```python
from build123d import *

# Parameters (mm, degrees)
SKETCH_1_R               = 1.65
SKETCH_1_R_2             = 9
EXTRUDE_1_DEPTH          = 3
SKETCH_2_R               = 15.5
SKETCH_2_R_2             = 9
EXTRUDE_2_DEPTH          = 7
SKETCH_3_W               = 2.5
SKETCH_3_H               = 20
CUT_EXTRUDE_1_DEPTH      = 28
CUT_EXTRUDE_2_DEPTH      = 44.016618519
CUT_EXTRUDE_2_DEPTH_BACK = 44.016618519
SKETCH_4_R               = 1.1
SKETCH_5_R               = 10
CUT_EXTRUDE_3_DEPTH      = 43.210780613
SKETCH_6_R               = 1.9
CUT_EXTRUDE_8_DEPTH      = 13
CHAMFER_1_SIZE           = 2
FILLET_2_R               = 2
SKETCH_7_R               = 4
SKETCH_7_R_2             = 1.65
EXTRUDE_3_DEPTH          = 2
FILLET_3_R               = 0.5


with BuildPart() as part:
    # 草图1 → 凸台-拉伸1 (new body)
    with BuildSketch(Plane.XY):
        Polygon((0, 31), (-26.846787517, -15.5), (26.846787517, -15.5), align=None)
        with Locations((0, 20)):
            Circle(SKETCH_1_R, mode=Mode.SUBTRACT)
        with Locations((17.320508076, -10)):
            Circle(SKETCH_1_R, mode=Mode.SUBTRACT)
        with Locations((-17.320508076, -10)):
            Circle(SKETCH_1_R, mode=Mode.SUBTRACT)
        Circle(SKETCH_1_R_2, mode=Mode.SUBTRACT)
    extrude(amount=EXTRUDE_1_DEPTH)

    # 草图2 → 凸台-拉伸2 (add)
    with BuildSketch(Plane.XY.offset(3)):
        with Locations(Location((0, 0, 0), (0, 0, 150))):
            Circle(SKETCH_2_R)
        Circle(SKETCH_2_R_2, mode=Mode.SUBTRACT)
    extrude(amount=EXTRUDE_2_DEPTH)

    # 草图3 → 切除-拉伸1 (cut)
    with BuildSketch(Plane.XY.offset(10)):
        with Locations((0, -9)):
            Rectangle(SKETCH_3_W, SKETCH_3_H)
    extrude(amount=-CUT_EXTRUDE_1_DEPTH, mode=Mode.SUBTRACT)

    # 草图4 → 切除-拉伸2 (cut, two sides: drawn at the far end of the back side and taken through both)
    with BuildSketch(Plane(origin=(-1.25, 0, 0), x_dir=(0, 0, -1), z_dir=(1, 0, 0)).offset(-CUT_EXTRUDE_2_DEPTH_BACK)):
        with Locations(Location((-8, -13, 0), (0, 0, 90))):
            Circle(SKETCH_4_R)
    extrude(amount=CUT_EXTRUDE_2_DEPTH + CUT_EXTRUDE_2_DEPTH_BACK, mode=Mode.SUBTRACT)

    # 草图5 → 切除-拉伸3 (cut, through all)
    with BuildSketch(Plane.XY.offset(10)):
        Circle(SKETCH_5_R)
    extrude(amount=-CUT_EXTRUDE_3_DEPTH, mode=Mode.SUBTRACT)

    # 草图6 → 切除-拉伸8 (cut)
    with BuildSketch(Plane(origin=(18.75, 0, 0), x_dir=(0, 0, -1), z_dir=(1, 0, 0))):
        with Locations((-8, -13)):
            Circle(SKETCH_6_R)
    cut_extrude_8 = extrude(amount=-CUT_EXTRUDE_8_DEPTH, mode=Mode.SUBTRACT)

    # 镜向1: 切除-拉伸8 across plane
    add(cut_extrude_8.mirror(Plane(origin=(0, 0, 0), x_dir=(0, 0, 1), z_dir=(1, 0, 0))), mode=Mode.SUBTRACT)

    # 倒角1
    # the kernel refuses this chamfer: 2 mm, written as the material it adds along each edge
    with BuildSketch(Plane(origin=(0, 0, 3), x_dir=(-0.24867915141291427, -0.9685859175378057, 0), z_dir=(-0.9685859175378057, 0.24867915141291427, 0))) as chamfer_1_piece_1_section:
        Polygon((15.5 + CHAMFER_1_SIZE, 0), (15.5, CHAMFER_1_SIZE), (15.5, 0), align=None)
    chamfer_1_piece_1 = revolve(axis=Axis((0, 0, 3), (0, 0, 1)), revolution_arc=134.399365049, mode=Mode.PRIVATE)
    chamfer_1_piece_1 = split(chamfer_1_piece_1, bisect_by=Plane(origin=(-1.25, -15.346279834, 3.925823909), z_dir=(-1, 0, 0)), keep=Keep.TOP, mode=Mode.PRIVATE)
    chamfer_1_piece_1 = split(chamfer_1_piece_1, bisect_by=Plane(origin=(-2.983750464, -15.5, 3.925823909), z_dir=(0, 1, 0)), keep=Keep.TOP, mode=Mode.PRIVATE)
    add(chamfer_1_piece_1)
    with BuildSketch(Plane(origin=(0, 0, 3), x_dir=(-0.24867915141291427, -0.9685859175378057, 0), z_dir=(-0.9685859175378057, 0.24867915141291427, 0))) as chamfer_1_piece_2_section:
        Polygon((15.5 + CHAMFER_1_SIZE, 0), (15.5, CHAMFER_1_SIZE), (15.5, 0), align=None)
    chamfer_1_piece_2 = revolve(axis=Axis((0, 0, 3), (0, 0, 1)), revolution_arc=134.399365049, mode=Mode.PRIVATE)
    chamfer_1_piece_2 = split(chamfer_1_piece_2, bisect_by=Plane(origin=(1.25, -7.656401186, 3.97388988), z_dir=(1, 0, 0)), keep=Keep.TOP, mode=Mode.PRIVATE)
    chamfer_1_piece_2 = split(chamfer_1_piece_2, bisect_by=Plane(origin=(14.586588654, -15.5, 3.97388988), z_dir=(0, 1, 0)), keep=Keep.TOP, mode=Mode.PRIVATE)
    chamfer_1_piece_2 = split(chamfer_1_piece_2, bisect_by=Plane(origin=(20.385359887, -4.308479054, 3.97388988), z_dir=(-0.8660254037844387, -0.5000000000000001, 0)), keep=Keep.TOP, mode=Mode.PRIVATE)
    add(chamfer_1_piece_2)
    with BuildSketch(Plane(origin=(0, 0, 3), x_dir=(-0.8660254037844386, 0.4999999999999999, 0), z_dir=(0.4999999999999999, 0.8660254037844386, 0))) as chamfer_1_piece_3_section:
        Polygon((15.5 + CHAMFER_1_SIZE, 0), (15.5, CHAMFER_1_SIZE), (15.5, 0), align=None)
    chamfer_1_piece_3 = revolve(axis=Axis((0, 0, 3), (0, 0, 1)), revolution_arc=134.399364936, mode=Mode.PRIVATE)
    chamfer_1_piece_3 = split(chamfer_1_piece_3, bisect_by=Plane(origin=(-20.385359891, -4.308479063, 3.973889878), z_dir=(0.8660254037844387, -0.5000000000000001, 0)), keep=Keep.TOP, mode=Mode.PRIVATE)
    chamfer_1_piece_3 = split(chamfer_1_piece_3, bisect_by=Plane(origin=(-1.25, -7.656401201, 3.973889878), z_dir=(-1, 0, 0)), keep=Keep.TOP, mode=Mode.PRIVATE)
    chamfer_1_piece_3 = split(chamfer_1_piece_3, bisect_by=Plane(origin=(-14.586588647, -15.5, 3.973889878), z_dir=(0, 1, 0)), keep=Keep.TOP, mode=Mode.PRIVATE)
    add(chamfer_1_piece_3)
    with BuildSketch(Plane(origin=(0, 0, 3), x_dir=(-0.8660254037844386, 0.4999999999999999, 0), z_dir=(0.4999999999999999, 0.8660254037844386, 0))) as chamfer_1_piece_4_section:
        Polygon((15.5 + CHAMFER_1_SIZE, 0), (15.5, CHAMFER_1_SIZE), (15.5, 0), align=None)
    chamfer_1_piece_4 = revolve(axis=Axis((0, 0, 3), (0, 0, 1)), revolution_arc=134.399364936, mode=Mode.PRIVATE)
    chamfer_1_piece_4 = split(chamfer_1_piece_4, bisect_by=Plane(origin=(1.25, -15.346279834, 3.925823908), z_dir=(1, 0, 0)), keep=Keep.TOP, mode=Mode.PRIVATE)
    chamfer_1_piece_4 = split(chamfer_1_piece_4, bisect_by=Plane(origin=(2.983750464, -15.5, 3.925823908), z_dir=(0, 1, 0)), keep=Keep.TOP, mode=Mode.PRIVATE)
    add(chamfer_1_piece_4)
    with BuildSketch(Plane(origin=(0, 0, 3), x_dir=(0.8660254027930385, 0.5000000017171554, 0), z_dir=(0.5000000017171554, -0.8660254027930385, 0))) as chamfer_1_piece_5_section:
        Polygon((15.5, CHAMFER_1_SIZE), (15.5 + CHAMFER_1_SIZE, 0), (15.5, 0), align=None)
    chamfer_1_piece_5 = revolve(axis=Axis((0, 0, 3), (0, 0, 1)), revolution_arc=119.999999886, mode=Mode.PRIVATE)
    chamfer_1_piece_5 = split(chamfer_1_piece_5, bisect_by=Plane(origin=(-6.289993318, 20.105411993, 3.973882667), z_dir=(0.8660254037844387, -0.5000000000000001, 0)), keep=Keep.TOP, mode=Mode.PRIVATE)
    chamfer_1_piece_5 = split(chamfer_1_piece_5, bisect_by=Plane(origin=(6.28999331, 20.105412007, 3.973882667), z_dir=(-0.8660254037844387, -0.5000000000000001, 0)), keep=Keep.TOP, mode=Mode.PRIVATE)
    add(chamfer_1_piece_5)

    # 圆角2
    fillet_2_edges = [part.edges().sort_by_distance(p)[0] for p in [
        (26.846787517, -15.5, 1.5),
        (-26.846787517, -15.5, 1.5),
        (0, 31, 1.5),
    ]]
    fillet(fillet_2_edges, radius=FILLET_2_R)

    # 草图7 → 凸台-拉伸3 (add)
    # profile 1 of 3: a face of its own
    with BuildSketch(Plane.XY.offset(3)):
        with Locations(Location((0, 20, 0), (0, 0, 223.309380883))):
            Circle(SKETCH_7_R)
        with Locations((0, 20)):
            Circle(SKETCH_7_R_2, mode=Mode.SUBTRACT)
    # profile 2 of 3: a face of its own
    with BuildSketch(Plane.XY.offset(3)):
        with Locations(Location((17.320508076, -10, 0), (0, 0, 196.690618915))):
            Circle(SKETCH_7_R)
        with Locations((17.320508076, -10)):
            Circle(SKETCH_7_R_2, mode=Mode.SUBTRACT)
    # profile 3 of 3: a face of its own
    with BuildSketch(Plane.XY.offset(3)):
        with Locations(Location((-17.320508076, -10, 0), (0, 0, 76.690618915))):
            Circle(SKETCH_7_R)
        with Locations((-17.320508076, -10)):
            Circle(SKETCH_7_R_2, mode=Mode.SUBTRACT)
    extrude(amount=EXTRUDE_3_DEPTH)

    # 圆角3
    # the kernel refuses this fillet: 0.5 mm, written as the material it adds along each edge
    with BuildSketch(Plane(origin=(-17.320508076, -10, 3), x_dir=(0.5191846053523372, 0.854662123628477, 0), z_dir=(0.854662123628477, -0.5191846053523372, 0))) as fillet_3_piece_1:
        with BuildLine():
            CenterArc((4 + FILLET_3_R, FILLET_3_R), FILLET_3_R, 180, 90)
            Line((4 + FILLET_3_R, 0), (4, 0))
            Line((4, 0), (4, FILLET_3_R))
        make_face()
    revolve(axis=Axis((-17.320508076, -10, 3), (0, 0, 1)), revolution_arc=302.555144431)
    with BuildSketch(Plane(origin=(17.320508076, -10, 3), x_dir=(-0.9997514133907861, 0.022295995674683326, 0), z_dir=(0.022295995674683326, 0.9997514133907861, 0))) as fillet_3_piece_2:
        with BuildLine():
            CenterArc((4 + FILLET_3_R, FILLET_3_R), FILLET_3_R, 180, 90)
            Line((4, FILLET_3_R), (4, 0))
            Line((4, 0), (4 + FILLET_3_R, 0))
        make_face()
    revolve(axis=Axis((17.320508076, -10, 3), (0, 0, 1)), revolution_arc=302.555144431)
    with BuildSketch(Plane(origin=(0, 20, 3), x_dir=(0.4805668111313066, -0.8769581176082967, 0), z_dir=(-0.8769581176082967, -0.4805668111313066, 0))) as fillet_3_piece_3:
        with BuildLine():
            CenterArc((4 + FILLET_3_R, FILLET_3_R), FILLET_3_R, 180, 90)
            Line((4 + FILLET_3_R, 0), (4, 0))
            Line((4, 0), (4, FILLET_3_R))
        make_face()
    revolve(axis=Axis((0, 20, 3), (0, 0, 1)), revolution_arc=302.555144229)


solid = part.part
```
Here's how the part is built. I have some questions about the finished solid (model axes, mm). A direction names the side the tool comes from. Give positions to 0.01 mm unless a question says otherwise; leave off trailing zeros. Loops run counter-clockwise (first coordinate to the right, second up) from the corner with the lowest first, then second, coordinate; pieces in that order, holes last. Notation, with made-up numbers: M -4,81.5 L 21,81.5 A14 ccw 21,85.5 Z; hole C -40,74 d3. An arc over 180 degrees is marked long. Put each result on its own line as item: value. Start each with the question number.
(1) I need wall thicknesses on line 1 along Y through (x, z) = (-1.5, 8); line 2 along Y through (x, z) = (1.5, 2); line 3 along Z through (x, y) = (-1, 26.5). Which ranges of each line are inside material? Lowest first, please. Write a range as [from, to].
(2) I want a section at B-B on z = 1.5. Please give me the cut outline in (x, y), then the cut area to 3 significant figures.
(3) For faces 4 (the flat face through (-5.75, -12, 7)), 5 (the flat face through (1.25, -13, 5)), 6 (the flat face through (-17, -8, 5)), 7 (the cylindrical face through (-3.53, -13.87, 7.33)), which set-ups out of +Z, -Z, +X, -X, +Y, -Y let a thin tool reach every point of the face, with its end or its side?
(4) If we mould it in two halves opening along Y, with no side actions, what happens to faces 1 (the flat face through (12, -15.5, 2)), 2 (the flat face through (17, -8, 5)), 3 (the conical face through (13.9, -7.55, 4.68))? For each: +Y half, -Y half, draft (parallel to the pull), parting line (faces both ways), or undercut.
(5) Will these pins go through, and if not, where does the flat tip stop? pin 1 Ø1.7 at (y, z) = (-12.5, 3.5) entering from +X; pin 2 Ø1.8 at (y, z) = (-13, 8) entering from +X; pin 3 Ø13 at (x, y) = (20.5, -9) entering from +Z; pin 4 Ø1.5 at (x, y) = (10, 15) entering from +Z.
(6) I want a section at A-A on x = 0. Please give me the cut outline in (y, z).
Answer block:
1. line 1: [-15.43, -14.1], [-11.9, -9.89], [9.89, 15.43]
1. line 2: [-15.5, -9.89], [9.89, 19.31], [20.69, 28.32]
1. line 3: [0, 3]
2. outline: M -25.11,-12.5 A2 ccw -23.38,-15.5 L -1.25,-15.5 L -1.25,-9.92 A10 cw long 1.25,-9.92 L 1.25,-15.5 L 23.38,-15.5 A2 ccw 25.11,-12.5 L 1.73,28 A2 ccw -1.73,28 Z; hole C -17.32,-10 d3.3; hole C 0,20 d3.3; hole C 17.32,-10 d3.3
2. area: 887 mm^2
3. face 4: -X
3. face 5: +Z, -Z, -Y
3. face 6: +Z, -X, -Y
3. face 7: +X, -X
4. face 1: -Y half
4. face 2: draft
4. face 3: undercut
5. pin 1: x = 25.36
5. pin 2: through
5. pin 3: z = 5
5. pin 4: z = 3.22
6. outline: M 10,0 L 18.35,0 L 18.35,5 L 16,5 L 16,4.5 L 15.5,5 L 15.5,10 L 10,10 Z; M 21.65,0 L 29,0 L 29,3 L 24.5,3 A0.5 cw 24,3.5 L 24,5 L 21.65,5 Z
